The model under review builds one solid part; all positions refer to its coordinate system, in mm. A direction names the side the tool comes from. Round coordinates to 2 decimals unless told otherwise and drop trailing zeros. Loops run counter-clockwise (first coordinate to the right, second up) from the corner with the lowest first, then second, coordinate; pieces in that order, holes last. Notation, with made-up numbers: M 63.25,24 L 88.25,24 A28 cw 88.25,61 Z; hole C 10,22.5 d7. An arc over 180 degrees is marked long. Answer as a JSON object with one key per item and string values. Group by question number.
Item 1: Insertion check: P1, Ø3, axis at x = 37.5, z = -2, coming from the +Y side; P2, Ø2, axis at x = 21, y = 4, coming from the +Z side; P3, Ø1.3, axis at x = 38, z = -2, coming from the -Y side. Each pin has a flat end and moves straight along its axis. Give the tip position at first contact, or say it passes through.
Item 2: Consider section A-A (z = -38). Give the boundary of the cut face in (x, y), and give its area (3 significant figures).
Item 3: Consider section D-D (y = 4.5). Give the boundary of the cut face in (x, z).
Item 4: The part is to be moulded in two halves that separate along Y. For faces 6 (the face through (37, 3, -3)), 7 (the face through (3.016, 1.479, -1.579)), 8 (the face through (6.104, 6, -3)), say which applies: +Y half, -Y half, draft (parallel to the pull), parting line (faces both ways), or undercut.
Item 5: Tool access review of faces 1 (the face through (3.945, 6.549, -3.86)), 2 (the face through (3.86, 6.549, -36.055)), 3 (the face through (36.14, 6.549, -3.945)), 4 (the face through (20, 9.287, -3)), 5 (the face through (36.055, 6.549, -36.14)): name each direction out of +Z, -Z, +X, -X, +Y, -Y from which nothing blocks a thin tool from reaching the whole face with its end or side.
Item 6: Consider section C-C (z = -2). Give the boundary of the cut face in (x, y).
Item 7: To check wall thickness, follow line 1 (X direction, y = 2.1, z = -38); line 2 (Z direction, x = 2, y = 1.3); line 3 (Y direction, x = 9, z = -4.5). State the ranges of each line that lie inside material, in increasing order.
Item 8: Consider section B-B (x = 31). Give the boundary of the cut face in (y, z).
```python
from build123d import *

# Parameters (mm, degrees)
SKETCH1_W           = 40
SKETCH1_H           = 40
SKETCH1_R           = 1.1
BOSS_EXTRUDE1_DEPTH = 10
CUT_EXTRUDE1_DEPTH  = 7
SKETCH3_W           = 27.571173344
SKETCH3_H           = 7.347922722
CUT_EXTRUDE2_DEPTH  = 7


with BuildPart() as part:
    # Sketch1 → Boss-Extrude1 (new body)
    with BuildSketch(Plane(origin=(0, 0, 0), x_dir=(1, 0, 0), z_dir=(0, 1, 0))):
        with Locations((20, 20)):
            Rectangle(SKETCH1_W, SKETCH1_H)
        with Locations((2, 38)):
            Circle(SKETCH1_R, mode=Mode.SUBTRACT)
        with Locations((38, 38)):
            Circle(SKETCH1_R, mode=Mode.SUBTRACT)
        with Locations((2, 2)):
            Circle(SKETCH1_R, mode=Mode.SUBTRACT)
        with Locations((38, 2)):
            Circle(SKETCH1_R, mode=Mode.SUBTRACT)
    extrude(amount=BOSS_EXTRUDE1_DEPTH)

    # Sketch2 → Cut-Extrude1 (cut)
    with BuildSketch(Plane(origin=(0, 10, 0), x_dir=(1, 0, 0), z_dir=(0, 1, 0))):
        with BuildLine():
            Line((0, 0), (5.519280972, 0))
            ThreePointArc((5.519280972, 0), (3.902721002, 3.902721002), (0, 5.519280972))
            Line((0, 5.519280972), (0, 0))
        make_face()
        with BuildLine():
            Line((40, 0), (40, 5.519280972))
            ThreePointArc((40, 5.519280972), (36.097278998, 3.902721002), (34.480719028, 0))
            Line((34.480719028, 0), (40, 0))
        make_face()
        with BuildLine():
            Line((40, 40), (34.480719028, 40))
            ThreePointArc((34.480719028, 40), (36.097278998, 36.097278998), (40, 34.480719028))
            Line((40, 34.480719028), (40, 40))
        make_face()
        with BuildLine():
            Line((0, 40), (0, 34.480719028))
            ThreePointArc((0, 34.480719028), (3.902721002, 36.097278998), (5.519280972, 40))
            Line((5.519280972, 40), (0, 40))
        make_face()
    extrude(amount=-CUT_EXTRUDE1_DEPTH, mode=Mode.SUBTRACT)

    # Sketch3 → Cut-Extrude2 (cut)
    with BuildSketch(Plane.XY):
        with Locations((19.889703926, 5.612775806)):
            Rectangle(SKETCH3_W, SKETCH3_H)
    extrude(amount=-CUT_EXTRUDE2_DEPTH, mode=Mode.SUBTRACT)


solid = part.part
```
Geometry results:
{
 "1": {"P1": "stops at y = 3", "P2": "stops at z = -7", "P3": "passes through"},
 "2": {"outline": "M 0,0 L 0.9,0 L 0.9,3 L 0,3 Z; M 3.1,0 L 36.9,0 L 36.9,3 L 34.86,3 L 34.86,10 L 5.14,10 L 5.14,3 L 3.1,3 Z; M 39.1,0 L 40,0 L 40,3 L 39.1,3 Z", "area": "315 mm^2"},
 "3": {"outline": "M 0,-34.48 A5.52 cw 5.52,-40 L 34.48,-40 A5.52 cw 40,-34.48 L 40,-5.52 A5.52 cw 34.48,0 L 33.68,0 L 33.68,-7 L 6.1,-7 L 6.1,0 L 5.52,0 A5.52 cw 0,-5.52 Z"},
 "4": {"face 6": "+Y half", "face 7": "draft", "face 8": "undercut"},
 "5": {"face 1": "+Z, -X, +Y", "face 2": "-Z, -X, +Y", "face 3": "+Z, +X, +Y", "face 4": "+Z", "face 5": "-Z, +X, +Y"},
 "6": {"outline": "M 0,0 L 0.9,0 L 0.9,3 L 0,3 Z; M 3.1,0 L 36.9,0 L 36.9,3 L 34.86,3 L 34.86,10 L 5.14,10 L 5.14,3 L 3.1,3 Z; M 39.1,0 L 40,0 L 40,3 L 39.1,3 Z; hole M 6.1,1.94 L 33.68,1.94 L 33.68,9.29 L 6.1,9.29 Z"},
 "7": {"line 1": "x = 0 to 0.9, 3.1 to 36.9, 39.1 to 40", "line 2": "z = -40 to -39.1, -36.9 to -3.1, -0.9 to 0", "line 3": "y = 0 to 1.94, 9.29 to 10"},
 "8": {"outline": "M 0,-40 L 10,-40 L 10,0 L 9.29,0 L 9.29,-7 L 1.94,-7 L 1.94,0 L 0,0 Z"}
}
